from build123d import *

# Parameters (mm, degrees)
BOSS_EXTRUDE1_DEPTH     = 61
CUT_EXTRUDE1_DEPTH      = 88.871376881
CUT_EXTRUDE1_DEPTH_BACK = 88.871376881
SKETCH2_R               = 3
FILLET1_R               = 3


with BuildPart() as part:
    # Sketch1 → Boss-Extrude1 (new body)
    with BuildSketch(Plane(origin=(0, 0, 0), x_dir=(1, 0, 0), z_dir=(0, 1, 0))):
        with BuildLine():
            Line((40, -51.75), (31.75, -51.75))
            ThreePointArc((31.75, -51.75), (0, -20), (-31.75, -51.75))
            Line((-31.75, -51.75), (-40, -51.75))
            Line((-40, -51.75), (-55, -51.75))
            Line((-55, -51.75), (-55, -41.75))
            Line((-55, -41.75), (-40, -41.75))
            ThreePointArc((-40, -41.75), (0, -10.518943744), (40, -41.75))
            Line((40, -41.75), (55, -41.75))
            Line((55, -41.75), (55, -51.75))
            Line((55, -51.75), (40, -51.75))
        make_face()
    extrude(amount=BOSS_EXTRUDE1_DEPTH)

    # Sketch2 → Cut-Extrude1 (cut, two sides: drawn at the far end of the back side and taken through both)
    with BuildSketch(Plane(origin=(0, 0, 41.75), x_dir=(-1, 0, 0), z_dir=(0, 0, -1)).offset(-CUT_EXTRUDE1_DEPTH_BACK)):
        with Locations((-47.5, 51)):
            Circle(SKETCH2_R)
        with Locations((-47.5, 10)):
            Circle(SKETCH2_R)
        with Locations((47.5, 10)):
            Circle(SKETCH2_R)
        with Locations((47.5, 51)):
            Circle(SKETCH2_R)
    extrude(amount=CUT_EXTRUDE1_DEPTH + CUT_EXTRUDE1_DEPTH_BACK, mode=Mode.SUBTRACT)

    # Fillet1
    fillet1_edges = [part.edges().sort_by_distance(p)[0] for p in [
        (-40, 30.5, 41.75),
        (40, 30.5, 41.75),
    ]]
    fillet(fillet1_edges, radius=FILLET1_R)


solid = part.part
Read the model definition and answer for the solid it produces. Units are mm, in the model's axes. A direction names the side the tool comes from. Give positions to 0.01 mm unless a question says otherwise; leave off trailing zeros. Write each loop counter-clockwise with the first axis right and the second up, starting at its lowest first coordinate (ties: lowest second). Pieces come first, ordered by that corner, then holes. Notation, with made-up numbers: M -28.75,53 L -9.75,53 A22 cw -9.75,81 Z; hole C 50,7.5 d4. An arc over 180 degrees is marked long. One line per item, written item: value. Start each with the question number.
(1) Find section A-A (x = -47.5). Determine the outline of the cut face in (y, z).
(2) Flat-ended cylindrical pins translate along their axes: pin 1 Ø12 at (x, y) = (-2.5, 34.5) entering from +Z; pin 2 Ø5 at (x, y) = (-47.5, 51) entering from +Z; pin 3 Ø10 at (x, y) = (46.5, 21) entering from -Z; pin 4 Ø6 at (x, y) = (-15.5, 11.5) entering from +Z. Find the tip coordinate at first contact, or state that the pin passes through.
(3) Determine the mould class of faces 3 (the flat face through (-55, 30, 47)), 4 (the cylindrical face through (0.698, 30.073, 20.008)), 5 (the cylindrical face through (47.891, 53.974, 46.82)), 6 (the flat face through (-49, 30, 41.75)) for opening direction X: pulls with the +X half, pulls with the -X half, needs draft (parallel to the pull), parting line crosses it, or undercut.
(4) Find section B-B (y = 10). Determine the outline of the cut face in (x, z).
(5) Find section C-C (z = 47.5). Determine the outline of the cut face in (x, y).
(6) A tool of negligible diameter and unlimited length cuts with its end or side. For faces 1 (the cylindrical face through (-40.52, 30.93, 41.18)), 2 (the flat face through (49, 30, 41.75)), from which of +Z, -Z, +X, -X, +Y, -Y can it reach the whole face along a straight path? Write none if from no direction.
(7) Find section D-D (y = 35). Determine the outline of the cut face in (x, z).
(8) Find the intervals of material crossed by line 1 (Y direction, x = 47.5, z = 45.25); line 2 (X direction, y = 51, z = 44); line 3 (X direction, y = 10, z = 45), in increasing order.
Results below:
1. outline: M 0,41.75 L 7,41.75 L 7,51.75 L 0,51.75 Z; M 13,41.75 L 48,41.75 L 48,51.75 L 13,51.75 Z; M 54,41.75 L 61,41.75 L 61,51.75 L 54,51.75 Z
2. pin 1: stops at z = 21.16
2. pin 2: passes through
2. pin 3: stops at z = 41.65
2. pin 4: stops at z = 25.95
3. face 3: pulls with the -X half
3. face 4: undercut
3. face 5: undercut
3. face 6: needs draft
4. outline: M -55,41.75 L -50.5,41.75 L -50.5,51.75 L -55,51.75 Z; M -44.5,41.75 L -42.28,41.75 A3 cw -39.41,39.63 A41.23 ccw 39.41,39.63 A3 cw 42.28,41.75 L 44.5,41.75 L 44.5,51.75 L 31.75,51.75 A31.75 cw -31.75,51.75 L -44.5,51.75 Z; M 50.5,41.75 L 55,41.75 L 55,51.75 L 50.5,51.75 Z
5. outline: M -55,0 L -31.46,0 L -31.46,61 L -55,61 Z; M 31.46,0 L 55,0 L 55,61 L 31.46,61 Z; hole C -47.5,10 d6; hole C -47.5,51 d6; hole C 47.5,10 d6; hole C 47.5,51 d6
6. face 1: -Z, -X, +Y, -Y
6. face 2: -Z, +X, +Y, -Y
7. outline: M -55,41.75 L -42.28,41.75 A3 cw -39.41,39.63 A41.23 ccw 39.41,39.63 A3 cw 42.28,41.75 L 55,41.75 L 55,51.75 L 31.75,51.75 A31.75 cw -31.75,51.75 L -55,51.75 Z
8. line 1: y = 0 to 7, 13 to 48, 54 to 61
8. line 2: x = -55 to -50.5, -44.5 to -30.79, 30.79 to 44.5, 50.5 to 55
8. line 3: x = -55 to -50.5, -44.5 to -31.02, 31.02 to 44.5, 50.5 to 55
